Geometry check sheet. Reference: the model listing, model coordinates, mm. Face numbers are marked on the shaded views. A direction names the side the tool comes from. Give positions to 0.01 mm unless a question says otherwise; leave off trailing zeros. Loops run counter-clockwise (first coordinate to the right, second up) from the corner with the lowest first, then second, coordinate; pieces in that order, holes last. Notation, with made-up numbers: (18.25, -25) - (58.25, -25) arc R23 ccw to (58.25, 2) - close; hole circle Ø5 at (66.25, -40). An arc over 180 degrees is marked (long way). Use a Markdown table: item, result. Add a question column.
1. Cross-section at D-D on y = -6.5. Enter the section's corners in (x, z).
2. Set-up check for the marked faces 1, 2 and 3: record each of +Z, -Z, +X, -X, +Y, -Y from which the full face is reachable in a straight line by a thin tool's end or side.
3. Cross-section at B-B on x = -19. Enter the section's corners in (y, z), and give its area (3 significant figures).
4. Material ranges on L1, parallel to X at y = 3, z = 2; L2, parallel to Z at x = -20.5, y = -4.5; L3, parallel to Z at x = 33, y = -11.5, recorded low to high.
5. Depth check by flat-ended pin: P1, Ø4.5, axis at x = 34, y = 11, coming from the -Z side; P2, Ø1.5, axis at y = -5.5, z = 7, coming from the +X side. Enter the tip coordinate at first touch or a pass-through.
6. Cross-section at A-A on y = 15.5. Enter the section's corners in (x, z).
7. Cross-section at C-C on z = 5.5. Enter the section's corners in (x, y), and give its area (3 significant figures).
from build123d import *

# Parameters (mm, degrees)
SKETCH1_W           = 65
SKETCH1_H           = 35
BOSS_EXTRUDE1_DEPTH = 12
SKETCH2_W           = 15
SKETCH2_H           = 35
CUT_EXTRUDE1_DEPTH  = 8
BOSS_EXTRUDE3_DEPTH = 20
CUT_EXTRUDE2_DEPTH  = 41


with BuildPart() as part:
    # Sketch1 → Boss-Extrude1 (new body)
    with BuildSketch(Plane.XY):
        with Locations((5.427350427, 2.767094017)):
            Rectangle(SKETCH1_W, SKETCH1_H)
    extrude(amount=BOSS_EXTRUDE1_DEPTH)

    # Sketch2 → Cut-Extrude1 (cut)
    with BuildSketch(Plane(origin=(0, 0, 0), x_dir=(-1, 0, 0), z_dir=(0, 0, -1))):
        with Locations((-30.427350427, 2.767094017)):
            Rectangle(SKETCH2_W, SKETCH2_H)
    extrude(amount=-CUT_EXTRUDE1_DEPTH, mode=Mode.SUBTRACT)

    # Sketch3 → Boss-Extrude3 (add)
    with BuildSketch(Plane.XY.offset(12)):
        Polygon((-27.072649573, 20.267094017), (-27.072649573, 10.267094017), (-2.072649573, -14.732905983), (37.927350427, -14.732905983), (37.927350427, 20.267094017), align=None)
    extrude(amount=BOSS_EXTRUDE3_DEPTH)

    # Sketch4 → Cut-Extrude2 (cut)
    with BuildSketch(Plane.XZ.offset(14.732905983)):
        Polygon((37.927350427, 32), (22.927350427, 32), (37.927350427, 17), align=None)
    extrude(amount=-CUT_EXTRUDE2_DEPTH, mode=Mode.SUBTRACT)


solid = part.part
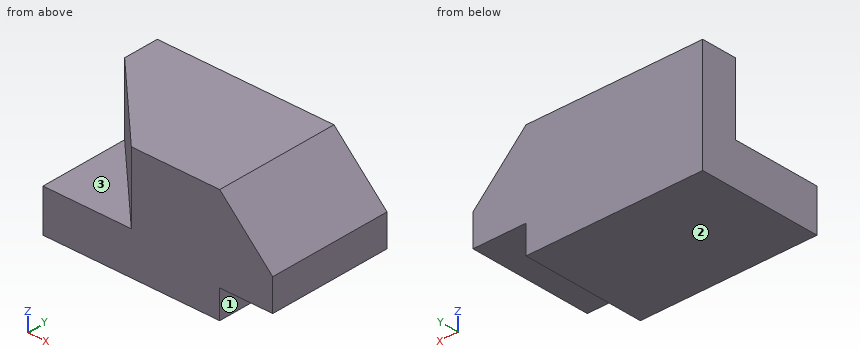
Values found:
| question | item | result |
|---|---|---|
| 1 | outline | (-27.07, 0) - (22.93, 0) - (22.93, 8) - (37.93, 8) - (37.93, 17) - (22.93, 32) - (-10.31, 32) - (-10.31, 12) - (-27.07, 12) - close |
| 2 | face 1 | -Z, +X, +Y, -Y |
| 2 | face 2 | -Z, +X, -X, +Y, -Y |
| 2 | face 3 | +Z, -X, -Y |
| 3 | outline | (-14.73, 0) - (20.27, 0) - (20.27, 32) - (2.19, 32) - (2.19, 12) - (-14.73, 12) - close |
| 3 | area | 781 mm2 |
| 4 | L1 | x = -27.07 to 22.93 |
| 4 | L2 | z = 0 to 12 |
| 4 | L3 | z = 8 to 21.93 |
| 5 | P1 | stops at z = 8 |
| 5 | P2 | stops at x = 22.93 |
| 6 | outline | (-27.07, 0) - (22.93, 0) - (22.93, 8) - (37.93, 8) - (37.93, 17) - (22.93, 32) - (-27.07, 32) - close |
| 7 | outline | (-27.07, -14.73) - (22.93, -14.73) - (22.93, 20.27) - (-27.07, 20.27) - close |
| 7 | area | 1,750 mm2 |
